Design review of the part built by this model. Coordinates are the model's own, in mm. Face numbers are marked on the shaded views. Coordinates: 2 decimals unless noted, no trailing zeros. Order: outer loops, then holes, each group sorted by start corner. A loop starts at its lowest first (then second) coordinate and runs counter-clockwise, first axis right, second up. Notation, with made-up numbers: (-4, -33) - (46, -33) arc R13 ccw to (46, -19) - close; hole circle Ø1 at (-36.5, 59). An arc over 180 degrees is marked (long way). Write each question's results on one line, items separated by ' | '. Start each with the question number.
```python
from build123d import *

# Parameters (mm, degrees)
IZIM1_R                     = 3
IZIM1_R_2                   = 6
Y_KSEKLIK_EKSTR_ZYON1_DEPTH = 10
KES_EKSTR_ZYON1_REACH       = 62
IZIM2_R                     = 1.5


with BuildPart() as part:
    # Çizim1 → Yükseklik-Ekstrüzyon1 (new body)
    with BuildSketch(Plane.XY):
        with BuildLine():
            Line((30, -14), (-25, -14))
            ThreePointArc((-25, -14), (-28.535533906, -12.535533906), (-30, -9))
            Line((-30, -9), (-30, 9))
            ThreePointArc((-30, 9), (-28.535533906, 12.535533906), (-25, 14))
            Line((-25, 14), (30, 14))
            Line((30, 14), (30, -14))
        make_face()
        with Locations((23, 7)):
            Circle(IZIM1_R, mode=Mode.SUBTRACT)
        with Locations((-19, 0)):
            Circle(IZIM1_R_2, mode=Mode.SUBTRACT)
        with Locations((9, -7)):
            Circle(IZIM1_R, mode=Mode.SUBTRACT)
    extrude(amount=Y_KSEKLIK_EKSTR_ZYON1_DEPTH)

    # Çizim2 → Kes-Ekstrüzyon1 (cut, up to next)
    with BuildSketch(Plane.ZY.offset(30), mode=Mode.PRIVATE) as kes_ekstr_zyon1_sk1:
        with Locations((5, 0)):
            Circle(IZIM2_R)
    kes_ekstr_zyon1_tool1 = extrude(kes_ekstr_zyon1_sk1.sketch, amount=-KES_EKSTR_ZYON1_REACH, mode=Mode.PRIVATE) & part.part
    add(kes_ekstr_zyon1_tool1.solids().sort_by_distance((-30, 0, 5))[0], mode=Mode.SUBTRACT)


solid = part.part
```
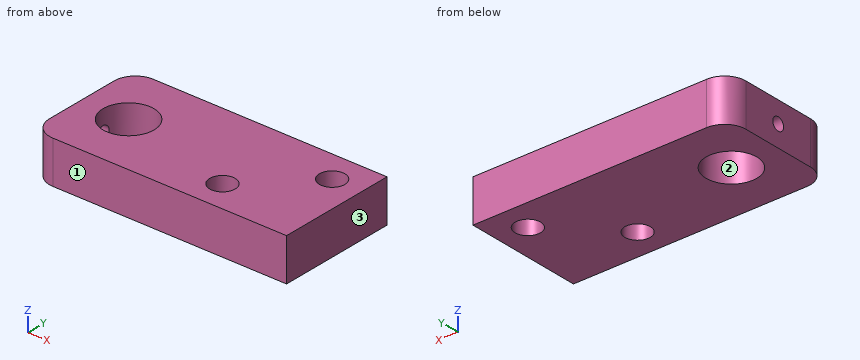
(1) Take a section at B-B (y = 7). State the section outline as (x, z) points.
(2) To check wall thickness, follow line 1 along X through (y, z) = (6.75, 3.5); line 2 along Y through (x, z) = (23, 2); line 3 along Y through (x, z) = (-19, 3.25). State the ranges of each line that lie inside material, in increasing order. Write a range as [from, to].
(3) Mouldability with a two-part tool opening along Y and no side actions: class the marked faces 1, 2 and 3 as +Y half, -Y half, draft (parallel to the pull), parting line (faces both ways), or undercut.
(4) Take a section at C-C (y = 0). State the section outline as (x, z) points.
(5) Take a section at D-D (z = 8.5). State the section outline as (x, y) points.
(6) Take a section at A-A (x = 23). State the section outline as (y, z) points, plus the area to 3 significant figures.
(7) Clearance check with a flat-ended pin moving along its axis: pin 1 (2.5 mm diameter, centred on y = 0, z = 5, fed in from -X). State where the tip first meets the part, or that it passes through.
Worked out:
1) outline: (-30, 0) - (20, 0) - (20, 10) - (-30, 10) - close; (26, 0) - (30, 0) - (30, 10) - (26, 10) - close
2) line 1: [-30, 20.01], [25.99, 30] | line 2: [-14, 4], [10, 14] | line 3: [-14, -6], [6, 14]
3) face 1: -Y half | face 2: undercut | face 3: draft
4) outline: (-30, 0) - (-25, 0) - (-25, 3.5) - (-30, 3.5) - close; (-30, 6.5) - (-25, 6.5) - (-25, 10) - (-30, 10) - close; (-13, 0) - (30, 0) - (30, 10) - (-13, 10) - close
5) outline: (-30, -9) arc R5 ccw to (-25, -14) - (30, -14) - (30, 14) - (-25, 14) arc R5 ccw to (-30, 9) - close; hole circle Ø12 at (-19, 0); hole circle Ø6 at (9, -7); hole circle Ø6 at (23, 7)
6) outline: (-14, 0) - (4, 0) - (4, 10) - (-14, 10) - close; (10, 0) - (14, 0) - (14, 10) - (10, 10) - close | area: 220 mm^2
7) pin 1: x = -13.13
